Input: dimensioned drawing with shaded views. Units: mm. Origin: part minimum x, y, z. Give positions to 0.01 mm unless a question says otherwise; leave off trailing zeros. Loops run counter-clockwise (first coordinate to the right, second up) from the corner with the lowest first, then second, coordinate; pieces in that order, holes last.
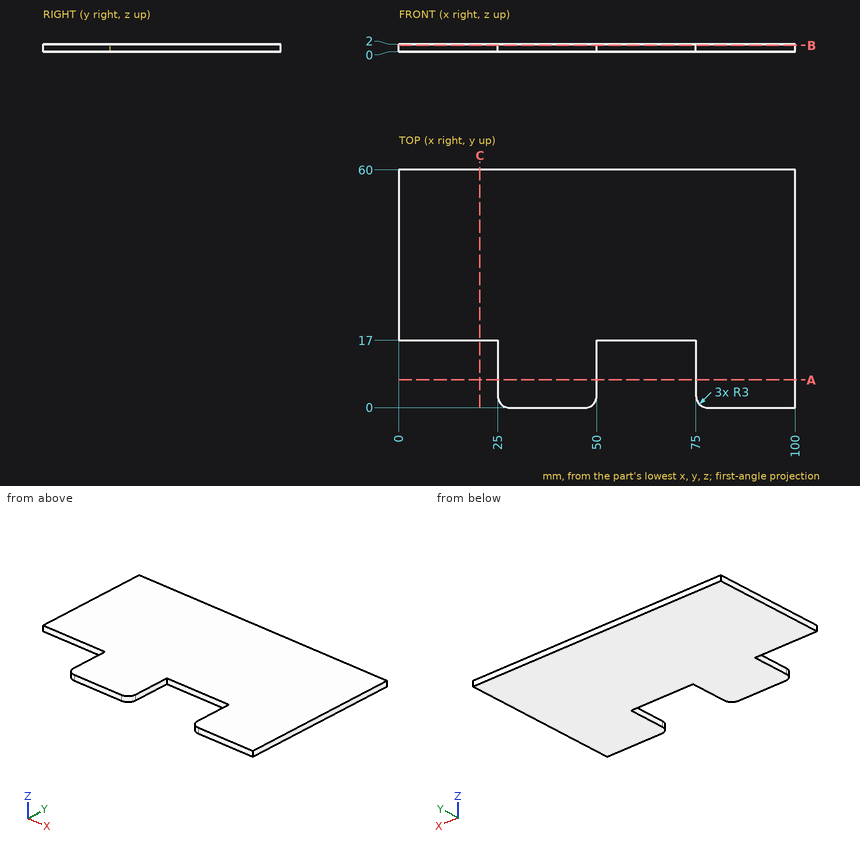
Item 1: Pin query (flat end, axial travel): pin 1 (1.5 mm diameter, centred on x = 52, y = 30.5, fed in from -Z); pin 2 (0.6 mm diameter, centred on y = 9, z = 1, fed in from -X); pin 3 (1 mm diameter, centred on x = 13.5, z = 1, fed in from -Y). Return the tip coordinate at first contact, or that it passes through.
Values follow:
pin 1: stops at z = 0
pin 2: stops at x = 25
pin 3: stops at y = 17
Item 2: Ray query, probe 1 along X at (y, z) = (12, 0.95); probe 2 along Y at (x, z) = (4, 1.75); probe 3 along Y at (x, z) = (76.5, 1.6). Return the intervals inside material, ascending.
Values follow:
probe 1: x = 25 to 50, 75 to 100
probe 2: y = 17 to 60
probe 3: y = 0.4 to 60
Item 3: Section query B-B on z = 1.65. Return loops of the section in (x, y), plus the area to 3 significant figures.
Values follow:
outline: (0, 17) - (25, 17) - (25, 3) arc R3 ccw to (28, 0) - (47, 0) arc R3 ccw to (50, 3) - (50, 17) - (75, 17) - (75, 3) arc R3 ccw to (78, 0) - (100, 0) - (100, 60) - (0, 60) - close
area: 5,140 mm2
Item 4: Section query C-C on x = 20.5. Return loops of the section in (y, z), plus the area to 3 significant figures.
Values follow:
outline: (17, 0) - (60, 0) - (60, 2) - (17, 2) - close
area: 86.0 mm2
Item 5: Section query A-A on y = 7. Return loops of the section in (x, z).
Values follow:
outline: (25, 0) - (50, 0) - (50, 2) - (25, 2) - close; (75, 0) - (100, 0) - (100, 2) - (75, 2) - close
